from build123d import *

# Parameters (mm, degrees)
FILLET1_R       = 0.6
FILLET2_R       = 1.2
HEX_2_DEPTH     = 6
THDSCHPAT_COUNT = 32
THDSCHPAT_PITCH = 1.7109375


with BuildPart() as part:
    # BodySke → Base-Revolve (revolve)
    with BuildSketch(Plane.XY, mode=Mode.PRIVATE) as base_revolve_sk:
        Polygon((0, 0), (0, 9), (12, 9), (12, 6), (71.036, 6), (72, 5.036), (72, 0), align=None)
    revolve(base_revolve_sk.sketch.rotate(Axis((-31.75, 0, 0), (1, 0, 0)), 90), axis=Axis((-31.75, 0, 0), (1, 0, 0)))  # turned: the seam where the file's is

    # Fillet1
    fillet1_edges = [part.edges().sort_by_distance(p)[0] for p in [
        (12, 0, -6),
    ]]
    fillet(fillet1_edges, radius=FILLET1_R)

    # Fillet2
    fillet2_edges = [part.edges().sort_by_distance(p)[0] for p in [
        (0, 0, -9),
    ]]
    fillet(fillet2_edges, radius=FILLET2_R)

    # Sketch2 → Hex-PreBroach (revolve, cut)
    with BuildSketch(Plane.XY, mode=Mode.PRIVATE) as hex_prebroach_sk:
        Polygon((0, 5.0125), (6, 5.0125), (8.893968224, 0), (0, 0), align=None)
    revolve(hex_prebroach_sk.sketch.rotate(Axis((0, 0, 0), (1, 0, 0)), 90), axis=Axis((0, 0, 0), (1, 0, 0)), mode=Mode.SUBTRACT)  # turned: the seam where the file's is

    # Sketch3 → Hex 2 (cut)
    with BuildSketch(Plane(origin=(0, 0, 0), x_dir=(0, 0.5, 0.866025404), z_dir=(-1, 0, 0))):
        Polygon((2.893968224, 5.0125), (-2.893968224, 5.0125), (-5.787936449, 0), (-2.893968224, -5.0125), (2.893968224, -5.0125), (5.787936449, 0), align=None)
    extrude(amount=-HEX_2_DEPTH, mode=Mode.SUBTRACT)

    # ThdSchSke → ThreadSchematic (revolve, cut)
    with BuildSketch(Plane.XY, mode=Mode.PRIVATE) as threadschematic_sk:
        Polygon((17.25, -5.036), (16.574999933, -6), (16.574999933, -7.5), (17.925000067, -7.5), (17.925000067, -6), align=None)
    threadschematic = revolve(threadschematic_sk.sketch.rotate(Axis((-3.175, 0, 0), (1, 0, 0)), 270), axis=Axis((-3.175, 0, 0), (1, 0, 0)), mode=Mode.SUBTRACT)  # turned: the seam where the file's is

    # ThdSchPat: ThreadSchematic ×32
    with Locations(*[(i * THDSCHPAT_PITCH, 0, 0) for i in range(1, THDSCHPAT_COUNT)]):
        add(threadschematic, mode=Mode.SUBTRACT)


solid = part.part
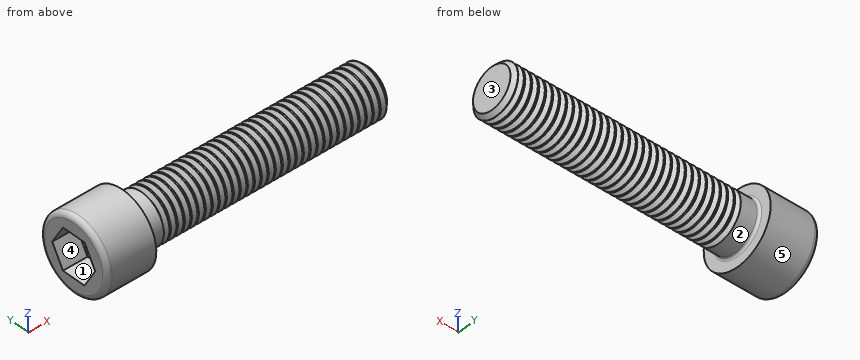
Could you check a few things on this model? Use its own coordinates, in mm. Face numbers are marked on the shaded views. A direction names the side the tool comes from. Give positions to 0.01 mm unless a question says otherwise; leave off trailing zeros. One line per item, written item: value. Start each with the question number.
1. Thinking about a two-plate mould opening in Z: for the marked faces 1, 2 and 3, which applies, +Z half, -Z half, draft (parallel to the pull), parting line (faces both ways), or undercut?
2. For the marked faces 4 and 5, which set-ups out of +Z, -Z, +X, -X, +Y, -Y let a thin tool reach every point of the face, with its end or its side?
3. For P1, Ø1.2, axis at y = -5, z = 0, coming from the -X side; P2, Ø3, axis at y = 1, z = 2, coming from the -X side; P3, Ø6, axis at x = 30, z = -5.5, coming from the +Y side, each with a flat end and sliding along its axis, tell me the tip position at first contact or that it passes through.
4. If I drill on probe 1 along X at (y, z) = (2.5, -6); probe 2 along Z at (x, y) = (20, -1.5); probe 3 along Y at (x, z) = (47, -3.25), over which ranges is the centre line in solid material (lowest first)?
Values:
1. face 1: undercut
1. face 2: parting line
1. face 3: draft
2. face 4: -X
2. face 5: +X, -X
3. P1: x = 6
3. P2: x = 6.74
3. P3: y = 5.45
4. probe 1: 0 to 12.01
4. probe 2: -5.8 to 5.8
4. probe 3: -5.02 to 5.02
